Design review of the part built by this model. Coordinates are the model's own, in mm. Face numbers are marked on the shaded views. Round coordinates to 2 decimals unless told otherwise and drop trailing zeros. Order: outer loops, then holes, each group sorted by start corner. A loop starts at its lowest first (then second) coordinate and runs counter-clockwise, first axis right, second up. Notation, with made-up numbers: (-9.5, 77.25) - (40.5, 77.25) arc R21 cw to (40.5, 100.25) - close; hole circle Ø7 at (67, 46). An arc over 180 degrees is marked (long way). Use CSV: the item, a comma, the result in double quotes. Start each with the question number.
from build123d import *

# Parameters (mm, degrees)
SKETCH_1_W          = 30
SKETCH_1_H          = 50
EXTRUDE_1_DEPTH     = 2
SKETCH_3_W          = 2
SKETCH_3_H          = 64
EXTRUDE_2_DEPTH     = 45
SKETCH_6_R          = 2.5
CUT_EXTRUDE_1_DEPTH = 3
SKETCH_7_R          = 2
EXTRUDE_4_DEPTH     = 4
SKETCH_8_R          = 0.75
EXTRUDE_5_DEPTH     = 5
FILLET_1_R          = 20
SKETCH_9_R          = 1.5
CUT_EXTRUDE_2_DEPTH = 31
SKETCH_10_W         = 20
SKETCH_10_H         = 8
EXTRUDE_6_DEPTH     = 5


with BuildPart() as part:
    # 草图1 → 凸台-拉伸1 (new body)
    with BuildSketch(Plane(origin=(0, 0, 0), x_dir=(1, 0, 0), z_dir=(0, 1, 0))):
        Rectangle(SKETCH_1_W, SKETCH_1_H)
    extrude(amount=-EXTRUDE_1_DEPTH)

    # 草图3 → 凸台-拉伸2 (add)
    with BuildSketch(Plane(origin=(0, 0, 0), x_dir=(1, 0, 0), z_dir=(0, 1, 0))):
        with Locations((-14, 0)):
            Rectangle(SKETCH_3_W, SKETCH_3_H)
    extrude(amount=EXTRUDE_2_DEPTH)

    # 草图6 → 切除-拉伸1 (cut, through all)
    with BuildSketch(Plane(origin=(-13, 0, 0), x_dir=(0, 0, -1), z_dir=(1, 0, 0))):
        with Locations((-28, 3)):
            Circle(SKETCH_6_R)
    extrude(amount=-CUT_EXTRUDE_1_DEPTH, mode=Mode.SUBTRACT)

    # 草图7 → 凸台-拉伸4 (add)
    with BuildSketch(Plane.ZY.offset(15)):
        with Locations((-18, 40)):
            Circle(SKETCH_7_R)
        with Locations((18, 40)):
            Circle(SKETCH_7_R)
        with Locations((-28, 3)):
            Circle(SKETCH_7_R)
    extrude(amount=EXTRUDE_4_DEPTH)

    # 草图8 → 凸台-拉伸5 (add)
    with BuildSketch(Plane.ZY.offset(19)):
        with Locations((-18, 40)):
            Circle(SKETCH_8_R)
        with Locations((18, 40)):
            Circle(SKETCH_8_R)
        with Locations((-28, 3)):
            Circle(SKETCH_8_R)
    extrude(amount=EXTRUDE_5_DEPTH)

    # 圆角1
    fillet_1_edges = [part.edges().sort_by_distance(p)[0] for p in [
        (-14, 45, 32),
        (-14, 45, -32),
    ]]
    fillet(fillet_1_edges, radius=FILLET_1_R)

    # 草图9 → 切除-拉伸2 (cut, through all)
    with BuildSketch(Plane.ZY.offset(15)):
        with Locations((-3, 22)):
            Circle(SKETCH_9_R)
        with Locations((3, 22)):
            Circle(SKETCH_9_R)
    extrude(amount=-CUT_EXTRUDE_2_DEPTH, mode=Mode.SUBTRACT)

    # 镜向1: part across plane


with BuildPart() as part_1:
    add(part.part)
    add(part.part.mirror(Plane.ZY))

    # 草图10 → 凸台-拉伸6 (add)
    with BuildSketch(Plane(origin=(0, 0, 0), x_dir=(1, 0, 0), z_dir=(0, 1, 0))):
        with Locations((0, 6)):
            Rectangle(SKETCH_10_W, SKETCH_10_H)
    extrude(amount=EXTRUDE_6_DEPTH)


solid = part_1.part
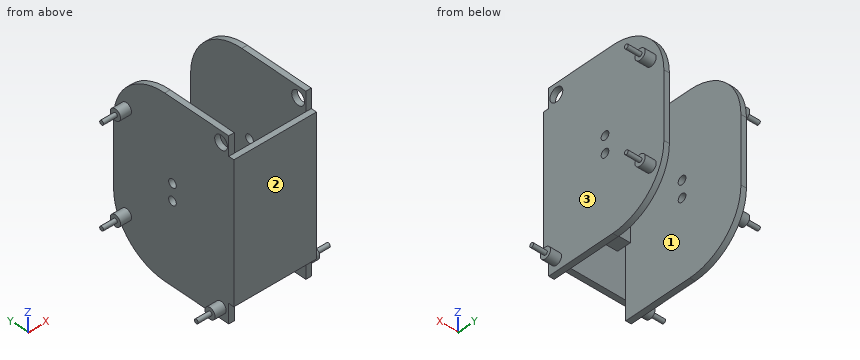
Q1. Take a section at D-D (z = 28). State the section outline as (x, y) points.
Q2. Take a section at B-B (y = 15). State the section outline as (x, z) points.
Q3. For L1, parallel to X at y = 19.5, z = -14.5; L2, parallel to Y at x = 14.45, z = -3; L3, parallel to Y at x = -4, z = -1.5, list the stretches that pass through material, from the lowest coordinate up. Write a range as [from, to].
Q4. The part is to be moulded in two halves that separate along X. For the marked faces 1, 2 and 3, say which applies: +X half, -X half, draft (parallel to the pull), parting line (faces both ways), or undercut.
Q5. Clearance check with flat-ended pins moving along their axes: pin 1 (1.6 mm diameter, centred on x = -5, y = -1, fed in from -Z); pin 2 (5 mm diameter, centred on y = 31.5, z = -13, fed in from -X); pin 3 (3 mm diameter, centred on y = 9.5, z = -21.5, fed in from +X); pin 4 (4 mm diameter, centred on x = 9.5, y = 13.5, fed in from -Z). State where each tip first meets the part, or that it passes through.
Q6. Take a section at A-A (z = -3). State the section outline as (x, y) points.
Q7. Take a section at C-C (x = -4). State the section outline as (y, z) points, plus the area to 3 significant figures.
Findings below:
1,outline,"(-15, 0) - (-13, 0) - (-13, 0.5) - (-15, 0.5) - close; (-15, 5.5) - (-13, 5.5) - (-13, 37) - (-15, 37) - close; (13, 0) - (15, 0) - (15, 0.5) - (13, 0.5) - close; (13, 5.5) - (15, 5.5) - (15, 37) - (13, 37) - close"
2,outline,"(-15, -32) - (-13, -32) - (-13, 32) - (-15, 32) - close; (13, -32) - (15, -32) - (15, 32) - (13, 32) - close"
3,L1,"x = [-15, -13], [13, 15]"
3,L2,"y = [-2, 20.5], [23.5, 45]"
3,L3,"y = [-2, 0]"
4,face 1,"undercut"
4,face 2,"draft"
4,face 3,"+X half"
5,pin 1,"stops at z = -25"
5,pin 2,"stops at x = -15"
5,pin 3,"stops at x = 15"
5,pin 4,"passes through"
6,outline,"(-15, -2) - (15, -2) - (15, 20.5) - (13, 20.5) - (13, 0) - (10, 0) - (10, 5) - (-10, 5) - (-10, 0) - (-13, 0) - (-13, 20.5) - (-15, 20.5) - close; (-15, 23.5) - (-13, 23.5) - (-13, 45) - (-15, 45) - close; (13, 23.5) - (15, 23.5) - (15, 45) - (13, 45) - close"
7,outline,"(-2, -25) - (0, -25) - (0, -10) - (5, -10) - (5, -2) - (0, -2) - (0, 25) - (-2, 25) - close"
7,area,"140 mm^2"
